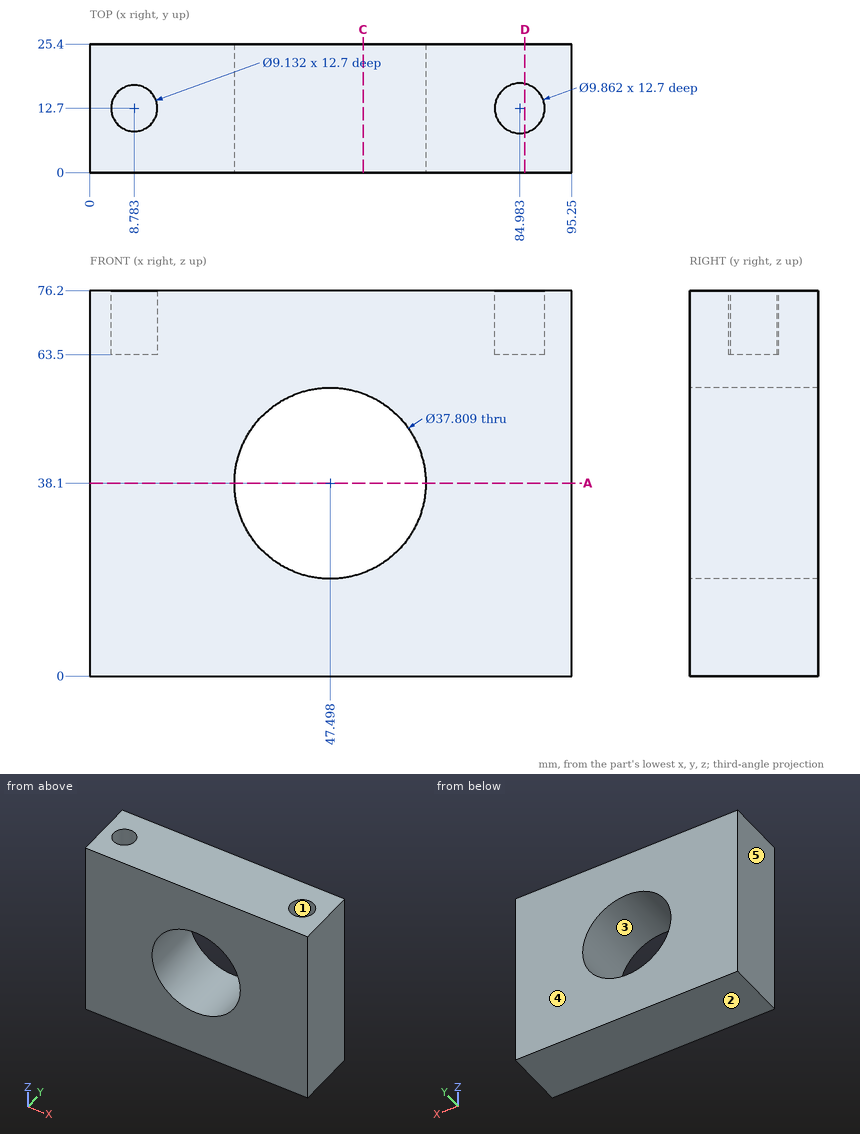
Check sheet for the drawn part. Datum: minimum x, y, z corner. Units: mm. A direction names the side the tool comes from. Round coordinates to 2 decimals unless told otherwise and drop trailing zeros. Order: outer loops, then holes, each group sorted by start corner. A loop starts at its lowest first (then second) coordinate and runs counter-clockwise, first axis right, second up. Notation, with made-up numbers: M -29,-12.75 L 13,-12.75 A17 ccw 13,4.25 Z; hole C 29,-37.75 d8. An arc over 180 degrees is marked long. Answer in a Markdown table with one row per item.
(1) Material ranges on line 1 along X through (y, z) = (10.5, 38.1); line 2 along Z through (x, y) = (59, 6.25) (1 decimal); line 3 along Z through (x, y) = (11, 12.75), recorded low to high. Write a range as from..to.
Findings:
| item | result |
|---|---|
| line 1 | x = 0..28.59, 66.4..95.25 |
| line 2 | z = 0..23.1, 53.1..76.2 |
| line 3 | z = 0..63.5 |
(2) Gauge pin test, flat end, axial feed: pin 1 (8 mm diameter, centred on x = 84.98, y = 12.7, fed in from +Z). Record the tip position at first contact, or that the pin passes through.
Findings:
| item | result |
|---|---|
| pin 1 | stops at z = 63.5 |
(3) Draft check along X on the marked faces 3, 4 and 5. Enter one of: +X half, -X half, draft (parallel to the pull), parting line (faces both ways), or undercut.
Findings:
| item | result |
|---|---|
| face 3 | undercut |
| face 4 | draft |
| face 5 | -X half |
(4) Section check A-A on z = 38.1. Record the boundary of the cut face in (x, y), plus the area to 3 significant figures.
Findings:
| item | result |
|---|---|
| outline | M 0,0 L 28.59,0 L 28.59,25.4 L 0,25.4 Z; M 66.4,0 L 95.25,0 L 95.25,25.4 L 66.4,25.4 Z |
| area | 1,460 mm^2 |
(5) Set-up check for the marked faces 1 and 2: record each of +Z, -Z, +X, -X, +Y, -Y from which the full face is reachable in a straight line by a thin tool's end or side.
Findings:
| item | result |
|---|---|
| face 1 | +Z |
| face 2 | -Z, +X, -X, +Y, -Y |
(6) Section check D-D on x = 86. Record the boundary of the cut face in (y, z) (1 decimal), plus the area to 3 significant figures.
Findings:
| item | result |
|---|---|
| outline | M 0,0 L 25.4,0 L 25.4,76.2 L 17.5,76.2 L 17.5,63.5 L 7.9,63.5 L 7.9,76.2 L 0,76.2 Z |
| area | 1,810 mm^2 |
(7) Section check C-C on x = 54. Record the boundary of the cut face in (y, z), plus the area to 3 significant figures.
Findings:
| item | result |
|---|---|
| outline | M 0,0 L 25.4,0 L 25.4,20.35 L 0,20.35 Z; M 0,55.85 L 25.4,55.85 L 25.4,76.2 L 0,76.2 Z |
| area | 1,030 mm^2 |
